Verification items for this drawing (mm, ordinates from the low corner). Round coordinates to 2 decimals unless told otherwise and drop trailing zeros. Loops run counter-clockwise (first coordinate to the right, second up) from the corner with the lowest first, then second, coordinate; pieces in that order, holes last. Notation, with made-up numbers: (74.5, 42) -> (124.5, 42) arc R34 ccw to (124.5, 78) -> close; hole circle Ø11 at (-5.75, 3.5). An arc over 180 degrees is marked (long way). One line per item, written item: value. Start each with the question number.
1. Release check for a two-part mould opening along X. For the marked faces 1, 2 and 3 record: +X half, -X half, draft (parallel to the pull), parting line (faces both ways), or undercut.
2. Material ranges on L1, parallel to Y at x = 22.5, z = 8.5; L2, parallel to X at y = 22.5, z = 6; L3, parallel to X at y = 22.5, z = 10.25, recorded low to high.
3. Go/stop test with flat-tipped pins: pin 1 (6 mm diameter, centred on y = 31, z = 2.5, fed in from -X); pin 2 (6 mm diameter, centred on x = 34, z = 4, fed in from -Y); pin 3 (5.5 mm diameter, centred on y = 23.5, z = 5, fed in from +X). Record where each tip stops, or that it passes through.
4. Cross-section at C-C on z = 12. Record the cut outline in (x, y).
5. Cross-section at D-D on x = 14.5. Record the cut outline in (y, z), then the cut area to 3 significant figures.
6. Cross-section at A-A on y = 22.5. Record the cut outline in (x, z), then the cut area to 3 significant figures.
7. Cross-section at B-B on x = 22.5. Record the cut outline in (y, z).
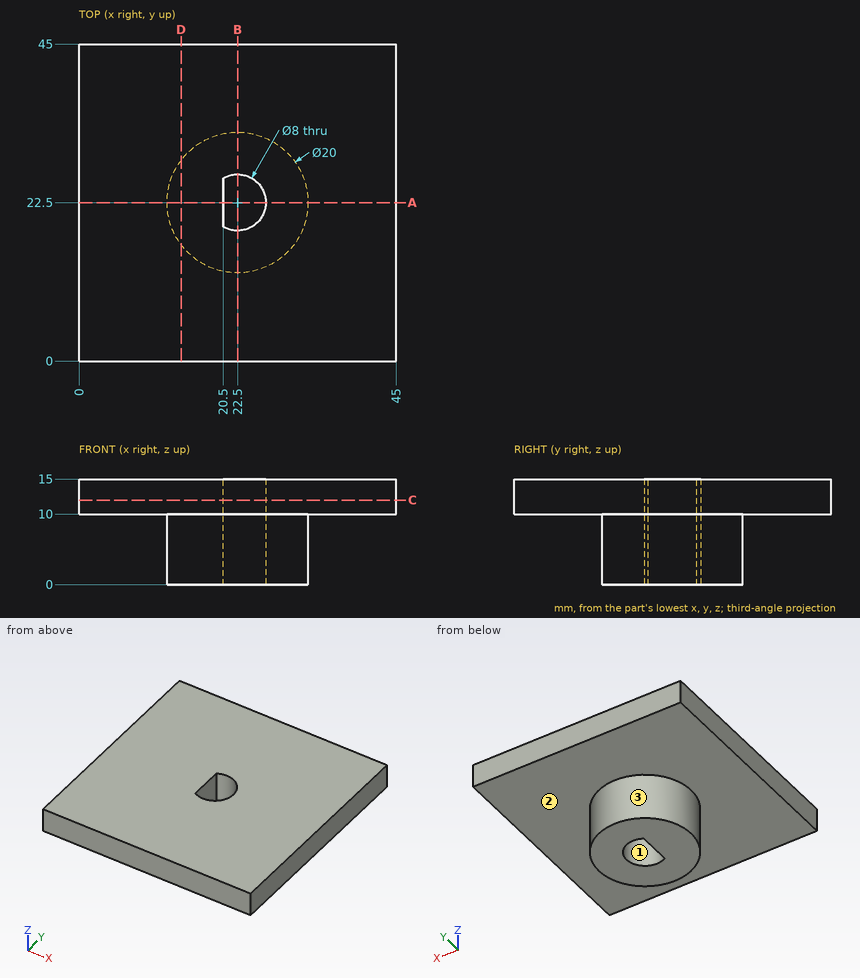
Taken from the geometry:
1. face 1: undercut
1. face 2: draft
1. face 3: parting line
2. L1: y = 12.5 to 18.5, 26.5 to 32.5
2. L2: x = 12.5 to 20.5, 26.5 to 32.5
2. L3: x = 0 to 20.5, 26.5 to 45
3. pin 1: stops at x = 14.15
3. pin 2: stops at y = 17.23
3. pin 3: stops at x = 32.5
4. outline: (0, 0) -> (45, 0) -> (45, 45) -> (0, 45) -> close; hole (20.5, 19.04) arc R4 ccw (long way) to (20.5, 25.96) -> close
5. outline: (0, 10) -> (16.5, 10) -> (16.5, 0) -> (28.5, 0) -> (28.5, 10) -> (45, 10) -> (45, 15) -> (0, 15) -> close
5. area: 345 mm2
6. outline: (0, 10) -> (12.5, 10) -> (12.5, 0) -> (20.5, 0) -> (20.5, 15) -> (0, 15) -> close; (26.5, 0) -> (32.5, 0) -> (32.5, 10) -> (45, 10) -> (45, 15) -> (26.5, 15) -> close
6. area: 335 mm2
7. outline: (0, 10) -> (12.5, 10) -> (12.5, 0) -> (18.5, 0) -> (18.5, 15) -> (0, 15) -> close; (26.5, 0) -> (32.5, 0) -> (32.5, 10) -> (45, 10) -> (45, 15) -> (26.5, 15) -> close
